from build123d import *

# Parameters (mm, degrees)
SKETCH1_R           = 2.4892
BOSS_EXTRUDE1_DEPTH = 3.175
FILLET1_R           = 6.35


with BuildPart() as part:
    # Sketch1 → Boss-Extrude1 (new, symmetric)
    # profile 1 of 2: a face of its own
    with BuildSketch(Plane.XY):
        with BuildLine():
            Line((60.325, 47.625), (31.75, 47.625))
            Line((31.75, 47.625), (31.75, 40.5892))
            ThreePointArc((31.75, 40.5892), (33.5101302, 39.8601302), (34.2392, 38.1))
            ThreePointArc((34.2392, 38.1), (33.5101302, 36.3398698), (31.75, 35.6108))
            Line((31.75, 35.6108), (31.75, 27.8892))
            ThreePointArc((31.75, 27.8892), (33.5101302, 27.1601302), (34.2392, 25.4))
            ThreePointArc((34.2392, 25.4), (33.5101302, 23.6398698), (31.75, 22.9108))
            Line((31.75, 22.9108), (31.75, 15.1892))
            ThreePointArc((31.75, 15.1892), (33.5101302, 14.4601302), (34.2392, 12.7))
            ThreePointArc((34.2392, 12.7), (33.5101302, 10.9398698), (31.75, 10.2108))
            Line((31.75, 10.2108), (31.75, 3.175))
            Line((31.75, 3.175), (60.325, 3.175))
            Line((60.325, 3.175), (60.325, 47.625))
        make_face()
        with Locations((44.45, 12.7)):
            Circle(SKETCH1_R, mode=Mode.SUBTRACT)
        with Locations((44.45, 25.4)):
            Circle(SKETCH1_R, mode=Mode.SUBTRACT)
        with Locations((44.45, 38.1)):
            Circle(SKETCH1_R, mode=Mode.SUBTRACT)
    # profile 2 of 2: a face of its own
    with BuildSketch(Plane.XY):
        with BuildLine():
            Line((31.75, 40.5892), (31.75, 47.625))
            Line((31.75, 47.625), (3.175, 47.625))
            Line((3.175, 47.625), (3.175, 3.175))
            Line((3.175, 3.175), (31.75, 3.175))
            Line((31.75, 3.175), (31.75, 10.2108))
            ThreePointArc((31.75, 10.2108), (29.2608, 12.7), (31.75, 15.1892))
            Line((31.75, 15.1892), (31.75, 22.9108))
            ThreePointArc((31.75, 22.9108), (29.2608, 25.4), (31.75, 27.8892))
            Line((31.75, 27.8892), (31.75, 35.6108))
            ThreePointArc((31.75, 35.6108), (29.2608, 38.1), (31.75, 40.5892))
        make_face()
        with Locations((19.05, 12.7)):
            Circle(SKETCH1_R, mode=Mode.SUBTRACT)
        with Locations((19.05, 25.4)):
            Circle(SKETCH1_R, mode=Mode.SUBTRACT)
        with Locations((19.05, 38.1)):
            Circle(SKETCH1_R, mode=Mode.SUBTRACT)
    extrude(amount=BOSS_EXTRUDE1_DEPTH, both=True)

    # Fillet1
    fillet1_edges = [part.edges().sort_by_distance(p)[0] for p in [
        (60.325, 47.625, 0),
        (60.325, 3.175, 0),
        (3.175, 3.175, 0),
        (3.175, 47.625, 0),
    ]]
    fillet(fillet1_edges, radius=FILLET1_R)


solid = part.part
Geometry: final body of the model. Coordinates: model frame, mm. Coordinates: 2 decimals unless noted, no trailing zeros. Write each loop counter-clockwise with the first axis right and the second up, starting at its lowest first coordinate (ties: lowest second). Pieces come first, ordered by that corner, then holes. Notation, with made-up numbers: (-8, -17) - (26, -17) arc R31 cw to (26, 17) - close; hole circle Ø7 at (31.25, 83.5). An arc over 180 degrees is marked (long way). Return JSON: item names as keys, results as strings.
Item 1: Section query C-C (y = 23.5). Output: boundary loops of the cut face in (x, z) (3 decimals).
Completed:
{"outline": "(3.175, -3.175) - (17.442, -3.175) - (17.442, 3.175) - (3.175, 3.175) - close; (20.658, -3.175) - (30.142, -3.175) - (30.142, 3.175) - (20.658, 3.175) - close; (33.358, -3.175) - (42.842, -3.175) - (42.842, 3.175) - (33.358, 3.175) - close; (46.058, -3.175) - (60.325, -3.175) - (60.325, 3.175) - (46.058, 3.175) - close"}
Item 2: Section query A-A (x = 19.05). Output: boundary loops of the cut face in (y, z) (3 decimals), and give its area (3 significant figures).
Completed:
{"outline": "(3.175, -3.175) - (10.211, -3.175) - (10.211, 3.175) - (3.175, 3.175) - close; (15.189, -3.175) - (22.911, -3.175) - (22.911, 3.175) - (15.189, 3.175) - close; (27.889, -3.175) - (35.611, -3.175) - (35.611, 3.175) - (27.889, 3.175) - close; (40.589, -3.175) - (47.625, -3.175) - (47.625, 3.175) - (40.589, 3.175) - close", "area": "187 mm2"}
Item 3: Section query B-B (z = 1.75). Count the separate pieces of the cut face and the enclosed holes in it, and give its area (3 significant figures).
Completed:
{"separate pieces": "1", "enclosed holes": "9", "area": "2,330 mm2"}
Item 4: Pin query (flat end, axial travel): pin 1 Ø3 at (x, y) = (44.45, 12.7) entering from -Z; pin 2 Ø8 at (x, y) = (44.45, 38.1) entering from -Z (3 decimals). Return the tip coordinate at first contact, or that it passes through.
Completed:
{"pin 1": "passes through", "pin 2": "stops at z = -3.175"}
Item 5: Line query: L1, parallel to Y at x = 44.45, z = 1.8 (3 decimals); L2, parallel to Y at x = 30.5, z = 2.5 (3 decimals); L3, parallel to X at y = 25, z = -0.75 (3 decimals). Output: solid intervals per line, ascending.
Completed:
{"L1": "y = 3.175 to 10.211, 15.189 to 22.911, 27.889 to 35.611, 40.589 to 47.625", "L2": "y = 3.175 to 10.547, 14.853 to 23.247, 27.553 to 35.947, 40.253 to 47.625", "L3": "x = 3.175 to 16.593, 21.507 to 29.293, 34.207 to 41.993, 46.907 to 60.325"}
